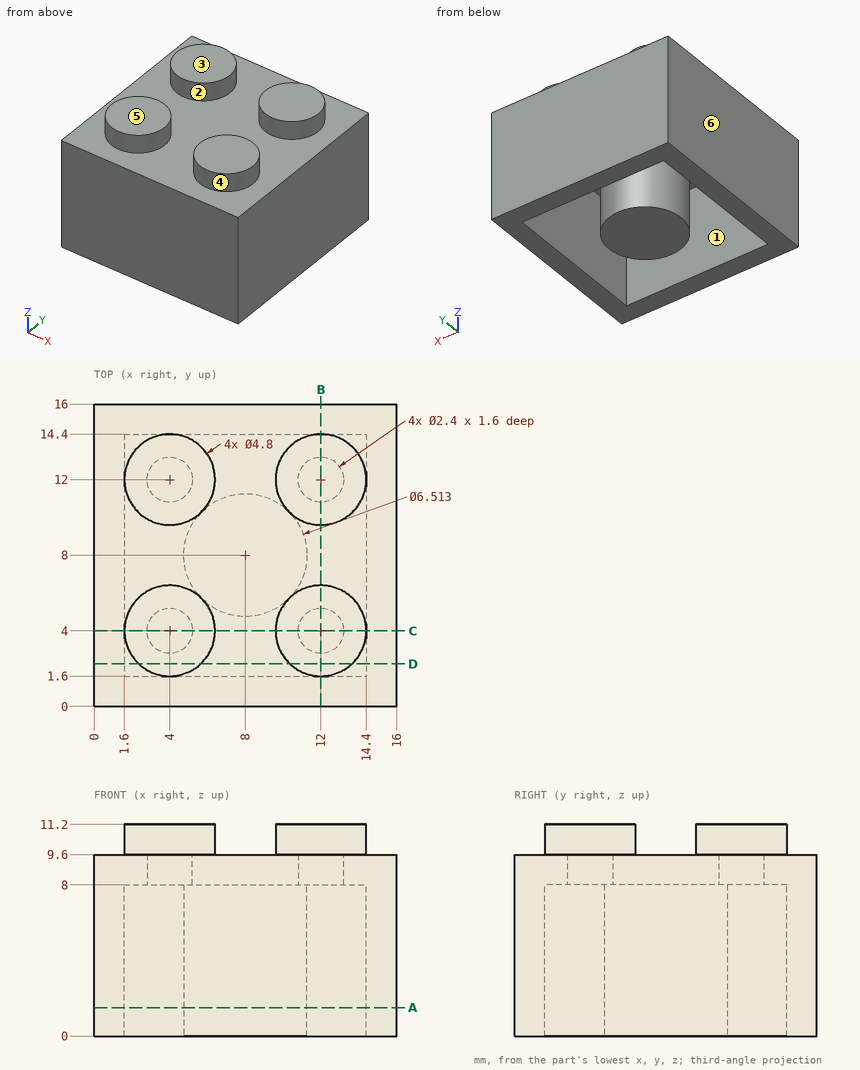
Geometry check sheet. Reference: drawing and pictorial views, mm from the part's lowest x, y, z. A direction names the side the tool comes from. Round coordinates to 2 decimals unless told otherwise and drop trailing zeros. Order: outer loops, then holes, each group sorted by start corner. A loop starts at its lowest first (then second) coordinate and runs counter-clockwise, first axis right, second up. Notation, with made-up numbers: (27.5, 51.5) - (64.5, 51.5) arc R35 cw to (64.5, 84.5) - close; hole circle Ø6 at (54.5, 71). An arc over 180 degrees is marked (long way). Write item = value, one per line.
Q1. Section check B-B (x = 12). Record the boundary of the cut face in (y, z).
Computed:
outline = (0, 0) - (1.6, 0) - (1.6, 8) - (2.8, 8) - (2.8, 9.6) - (5.2, 9.6) - (5.2, 8) - (10.8, 8) - (10.8, 9.6) - (13.2, 9.6) - (13.2, 8) - (14.4, 8) - (14.4, 0) - (16, 0) - (16, 9.6) - (14.4, 9.6) - (14.4, 11.2) - (9.6, 11.2) - (9.6, 9.6) - (6.4, 9.6) - (6.4, 11.2) - (1.6, 11.2) - (1.6, 9.6) - (0, 9.6) - close
Q2. Section check D-D (y = 2.25). Record the boundary of the cut face in (x, z).
Computed:
outline = (0, 0) - (1.6, 0) - (1.6, 8) - (14.4, 8) - (14.4, 0) - (16, 0) - (16, 9.6) - (13.64, 9.6) - (13.64, 11.2) - (10.36, 11.2) - (10.36, 9.6) - (5.64, 9.6) - (5.64, 11.2) - (2.36, 11.2) - (2.36, 9.6) - (0, 9.6) - close
Q3. Section check A-A (z = 1.5). Record the boundary of the cut face in (x, y).
Computed:
outline = (0, 0) - (16, 0) - (16, 16) - (0, 16) - close; circle Ø6.51 at (8, 8); hole (1.6, 1.6) - (14.4, 1.6) - (14.4, 14.4) - (1.6, 14.4) - close
Q4. Draft check along X on the marked faces 4, 5 and 6. Enter one of: pulls with the +X half, pulls with the -X half, needs draft (parallel to the pull), parting line crosses it, or undercut.
Computed:
face_4 = undercut
face_5 = needs draft
face_6 = pulls with the -X half
Q5. Thickness scan on line 1 along Y through (x, z) = (4, 8.3); line 2 along Y through (x, z) = (3, 1). Record the ranges inside material, lowest first.
Computed:
line_1 = 0 to 2.8, 5.2 to 10.8, 13.2 to 16
line_2 = 0 to 1.6, 14.4 to 16
Q6. Go/stop test with flat-tipped pins: pin 1 (1 mm diameter, centred on x = 7, y = 11, fed in from +Z); pin 2 (0.7 mm diameter, centred on x = 4, y = 12.5, fed in from -Z); pin 3 (2.5 mm diameter, centred on x = 12, y = 4, fed in from -Z). Record where each tip stops, or that it passes through.
Computed:
pin_1 = 9.6
pin_2 = 9.6
pin_3 = 8
Q7. Tool access check on the marked faces 1, 2 and 3. Record the directions out of +Z, -Z, +X, -X, +Y, -Y that give a thin tool (end or side, any length) a straight path to the whole face; none if there is none.
Computed:
face_1 = -Z
face_2 = +Z
face_3 = +Z, +X, -X, +Y, -Y
